Autodesk Inventor part; units mm, degrees
ref_plane "YZ Plane" through (0, 0, 0) normal (1, 0, 0) x (0, 1, 0)
ref_plane "XZ Plane" through (0, 0, 0) normal (0, 1, 0) x (-1, 0, 0)
ref_plane "XY Plane" through (0, 0, 0) normal (0, 0, 1) x (1, 0, 0)
sketch "Sketch1" plane through (0, 0, 0) normal (0, 1, 0) x (-1, 0, 0)
  line L0 (5, 0) -> (145, 0)
  line L1 (150, -5) -> (150, -145)
  line L2 (145, -150) -> (5, -150)
  line L3 (0, -145) -> (0, -5)
  arc A0 (150, -5) -> (145, 0) centre (145, -5) ccw
  arc A1 (150, -5) -> (145, 0) centre (145, -5) ccw
  arc A2 (145, -150) -> (150, -145) centre (145, -145) ccw
  arc A3 (5, 0) -> (0, -5) centre (5, -5) ccw
  arc A4 (0, -145) -> (5, -150) centre (5, -145) ccw
  circle A5 centre (128.033, -21.967) radius 9.5
  circle A6 centre (128.033, -128.033) radius 9.5
  circle A7 centre (21.967, -128.033) radius 9.5
  circle A8 centre (21.967, -21.967) radius 9.5
  circle A9 centre (21.967, -75) radius 5
  point P0 (150, -150)
  point P1 (150, 0)
  point P2 (0, -150)
  dimension "d12" = 150
  dimension "d13" = 150
  dimension "d22" = 5
  dimension "d23" = 5
  dimension "d28" = 19
  dimension "d29" = 19
  dimension "d30" = 19
  dimension "d31" = 19
  dimension "d32" = 10
extrude "Extrusion1" add sketch "Sketch1" along normal blind 6
sketch "Sketch2" plane through (0, 6, 0) normal (0, 1, 0) x (1, 0, 0)
  circle A0 centre (-128.033, 21.967) radius 9.5
  circle A1 centre (-21.967, 128.033) radius 9.5
  circle A2 centre (-128.033, 128.033) radius 9.5
  circle A3 centre (-75, 75) radius 3
  circle A4 centre (-21.967, 21.967) radius 9.5
  circle A5 centre (-106.8198, 43.1802) radius 2
  circle A6 centre (-43.1802, 43.1802) radius 2
  circle A7 centre (-43.1802, 106.8198) radius 2
  circle A8 centre (-106.8198, 106.8198) radius 2
  point P0 (0, 0)
  dimension "d35" = 6
  dimension "d40" = 4
  dimension "d41" = 4
  dimension "d42" = 4
  dimension "d43" = 4
  dimension "d47" = 30
extrude "Extrusion2" cut sketch "Sketch2" against normal blind 6 contours A3 | A5 | A6 | A7 | A8
sketch "Sketch3" plane through (0, 6, 0) normal (0, 1, 0) x (1, 0, 0)
  arc A0 (-5, 0) -> (0, 5) centre (-5, 5) ccw
  line L0 (-5, 0) -> (25, 0)
  line L1 (30, 5) -> (30, 145)
  line L2 (25, 150) -> (-5, 150)
  line L3 (-5, 150) -> (-5, 0)
  arc A1 (25, 0) -> (30, 5) centre (25, 5) ccw
  arc A2 (30, 145) -> (25, 150) centre (25, 145) ccw
  point P0 (0, 0)
  point P1 (30, 150)
  point P2 (30, 0)
  dimension "d48" = 35
  dimension "d49" = 150
  dimension "d50" = 5
extrude "Extrusion3" add sketch "Sketch3" against normal blind 6
sketch "Sketch4" plane through (0, 6, 0) normal (0, 1, 0) x (1, 0, 0)
  line L0 (30, 5) -> (30, 145)
  circle A0 centre (15, 55) radius 2.1
  circle A1 centre (15, 95) radius 2.1
  line L1 (-3, 80) -> (3, 80)
  line L2 (3, 80) -> (3, 90)
  line L3 (3, 90) -> (-3, 90)
  line L4 (-3, 90) -> (-3, 80)
  line L5 (-3, 70) -> (3, 70)
  line L6 (3, 70) -> (3, 60)
  line L7 (3, 60) -> (-3, 60)
  line L8 (-3, 60) -> (-3, 70)
  line L9 (15, 75) -> (15, 55)
  line L10 (15, 75) -> (15, 95)
  point P0 (0, 0)
  dimension "d55" = 4.2
  dimension "d56" = 4.2
  dimension "d58" = 10
  dimension "d60" = 6
  dimension "d61" = 10
  dimension "d62" = 6
  dimension "d63" = 10
  dimension "d67" = 20
  dimension "d68" = 20
extrude "Extrusion4" cut sketch "Sketch4" against normal blind 6
properties part number "E_base1"
Input: part model. Units: mm. Frame: model coordinates. A direction names the side the tool comes from. Coordinates: 2 decimals unless noted, no trailing zeros. Loops run counter-clockwise (first coordinate to the right, second up) from the corner with the lowest first, then second, coordinate; pieces in that order, holes last. Notation, with made-up numbers: (72, -5) - (92, -5) arc R23 cw to (92, 33) - close; hole circle Ø9 at (54, 69.5). An arc over 180 degrees is marked (long way). Answer in a Markdown table with one row per item.
(1) Cut plane D-D on x = -15. Output: boundary loops of the cut face in (y, z).
Model answer:
| item | result |
|---|---|
| outline | (0, -150) - (6, -150) - (6, -134.49) - (0, -134.49) - close; (0, -121.57) - (6, -121.57) - (6, -28.43) - (0, -28.43) - close; (0, -15.51) - (6, -15.51) - (6, 0) - (0, 0) - close |
(2) Cut plane C-C on z = -75. Output: boundary loops of the cut face in (x, y).
Model answer:
| item | result |
|---|---|
| outline | (-150, 0) - (-78, 0) - (-78, 6) - (-150, 6) - close; (-72, 0) - (-26.97, 0) - (-26.97, 6) - (-72, 6) - close; (-16.97, 0) - (30, 0) - (30, 6) - (-16.97, 6) - close |
(3) Pin query (flat end, axial travel): P1, Ø15, axis at x = -21.967, z = -21.967, coming from the +Y side. Return the tip coordinate at first contact, or that it passes through.
Model answer:
| item | result |
|---|---|
| P1 | passes through |
(4) Cut plane B-B on x = -75. Output: boundary loops of the cut face in (y, z).
Model answer:
| item | result |
|---|---|
| outline | (0, -150) - (6, -150) - (6, -78) - (0, -78) - close; (0, -72) - (6, -72) - (6, 0) - (0, 0) - close |
(5) Cut plane A-A on z = -55. Output: boundary loops of the cut face in (x, y), plus the area to 3 significant figures.
Model answer:
| item | result |
|---|---|
| outline | (-150, 0) - (12.9, 0) - (12.9, 6) - (-150, 6) - close; (17.1, 0) - (30, 0) - (30, 6) - (17.1, 6) - close |
| area | 1,050 mm² |
(6) Set-up query: faces 4 (the face through (-150, 3, -74)), 5 (the face through (3, 3, -85)). Return all of +Z, -Z, +X, -X, +Y, -Y with unobstructed straight access to the full face (end or side cutting, diameter ignored); none if empty.
Model answer:
| item | result |
|---|---|
| face 4 | +Z, -Z, -X, +Y, -Y |
| face 5 | +Y, -Y |
(7) Material intervals for L1, parallel to Z at x = 15, y = 4.1; L2, parallel to Z at x = 1, y = 0.75; L3, parallel to Z at x = -75, y = 2, sorted ascending. Write a range as from..to.
Model answer:
| item | result |
|---|---|
| L1 | z = -150..-97.1, -92.9..-57.1, -52.9..0 |
| L2 | z = -150..-90, -80..-70, -60..0 |
| L3 | z = -150..-78, -72..0 |
(8) Mould query, pull axis Z, two halves, no side actions, for faces 1 (the face through (-104.91, 3.04, -43.78)), 2 (the face through (30, 3, -74)), 3 (the face through (28, 3, -1)). Classes: pulls with the +Z half, pulls with the -Z half, needs draft (parallel to the pull), parting line crosses it, or undercut.
Model answer:
| item | result |
|---|---|
| face 1 | undercut |
| face 2 | needs draft |
| face 3 | pulls with the +Z half |
